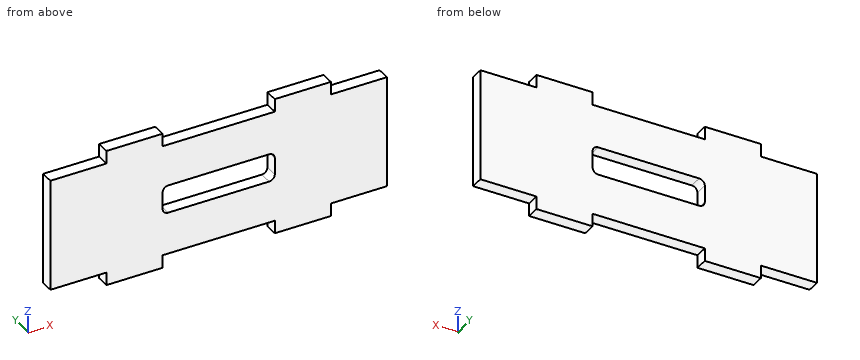
```python
from build123d import *

# Parameters (mm, degrees)
BOSS_EXTRUDE1_DEPTH = 2.3
SKETCH2_W           = 20
SKETCH2_H           = 5
CUT_EXTRUDE1_DEPTH  = 10
FILLET1_R           = 1


with BuildPart() as part:
    # Sketch1 → Boss-Extrude1 (new body)
    with BuildSketch(Plane(origin=(0, 0, 0), x_dir=(1, 0, 0), z_dir=(0, 1, 0))):
        Polygon((0, 0), (0, 20), (10, 20), (10, 22.3), (20, 22.3), (20, 20), (40, 20), (40, 22.3), (50, 22.3), (50, 20), (60, 20), (60, 0), (50, 0), (50, -2.3), (40, -2.3), (40, 0), (20, 0), (20, -2.3), (10, -2.3), (10, 0), align=None)
    extrude(amount=BOSS_EXTRUDE1_DEPTH)

    # Sketch2 → Cut-Extrude1 (cut)
    with BuildSketch(Plane(origin=(0, 2.3, 0), x_dir=(1, 0, 0), z_dir=(0, 1, 0))):
        with Locations((30, 10)):
            Rectangle(SKETCH2_W, SKETCH2_H)
    extrude(amount=-CUT_EXTRUDE1_DEPTH, mode=Mode.SUBTRACT)

    # Fillet1
    fillet1_edges = [part.edges().sort_by_distance(p)[0] for p in [
        (20, 1.15, -12.5),
        (40, 1.15, -12.5),
        (40, 1.15, -7.5),
        (20, 1.15, -7.5),
    ]]
    fillet(fillet1_edges, radius=FILLET1_R)


solid = part.part
```
For this review, take the finished solid that the model builds, in its own axes (mm). Coordinates: 2 decimals unless noted, no trailing zeros. Loops run counter-clockwise (first coordinate to the right, second up) from the corner with the lowest first, then second, coordinate; pieces in that order, holes last.
1. Add section D-D, the plane x = 51. Give the boundary of the cut face in (y, z).
2. Insertion check: P1, Ø0.7, axis at x = 30.5, y = 1.5, coming from the -Z side; P2, Ø1, axis at x = 7.5, y = 0.5, coming from the +Z side; P3, Ø1.2, axis at y = 1.5, z = 1.5, coming from the +X side. Each pin has a flat end and moves straight along its axis. Give the tip position at first contact, or say it passes through.
3. Add section C-C, the plane x = 33. Give the boundary of the cut face in (y, z).
4. Add section A-A, the plane z = 0.75. Give the boundary of the cut face in (x, y), then the cut area to 3 significant figures.
5. Add section B-B, the plane y = 1.55. Give the boundary of the cut face in (x, z), then the cut area to 3 significant figures.
6. For line 1 (Z direction, x = 26.5, y = 1.9); line 2 (X direction, y = 1.05, z = 1); line 3 (Z direction, x = 5, y = 1.3), list the stretches that pass through material, from the lowest coordinate up.
Result:
1. outline: (0, -20) - (2.3, -20) - (2.3, 0) - (0, 0) - close
2. P1: stops at z = -20
2. P2: stops at z = 0
2. P3: stops at x = 50
3. outline: (0, -20) - (2.3, -20) - (2.3, -12.5) - (0, -12.5) - close; (0, -7.5) - (2.3, -7.5) - (2.3, 0) - (0, 0) - close
4. outline: (10, 0) - (20, 0) - (20, 2.3) - (10, 2.3) - close; (40, 0) - (50, 0) - (50, 2.3) - (40, 2.3) - close
4. area: 46.0 mm2
5. outline: (0, -20) - (10, -20) - (10, -22.3) - (20, -22.3) - (20, -20) - (40, -20) - (40, -22.3) - (50, -22.3) - (50, -20) - (60, -20) - (60, 0) - (50, 0) - (50, 2.3) - (40, 2.3) - (40, 0) - (20, 0) - (20, 2.3) - (10, 2.3) - (10, 0) - (0, 0) - close; hole (20, -11.5) arc R1 ccw to (21, -12.5) - (39, -12.5) arc R1 ccw to (40, -11.5) - (40, -8.5) arc R1 ccw to (39, -7.5) - (21, -7.5) arc R1 ccw to (20, -8.5) - close
5. area: 1,190 mm2
6. line 1: z = -20 to -12.5, -7.5 to 0
6. line 2: x = 10 to 20, 40 to 50
6. line 3: z = -20 to 0
